```python
from build123d import *

# Parameters (mm, degrees)
F1_DEPTH = 1
F2_R     = 1.6
F3_DEPTH = 1.001
F4_R     = 0.5
F5_DEPTH = 1.001
F7_DEPTH = 1.001


with BuildPart() as f1:
    # F0 (on Front) → F1 (new body)
    with BuildSketch(Plane.XZ):
        Polygon((2, 30), (0, 30), (0, 0), (2, 0), (2, -1.3), (7, -1.3), (7, 0), (13, 0), (13, -1.3), (18, -1.3), (18, 0), (25, 0), (25, 30), (18, 30), (18, 31.3), (13, 31.3), (13, 30), (7, 30), (7, 31.3), (2, 31.3), align=None)
    extrude(amount=F1_DEPTH)

    # F2 (on face) → F3 (cut, through all)
    with BuildSketch(Plane.XZ.offset(1)):
        with Locations((10, 14)):
            Circle(F2_R)
        with BuildLine():
            ThreePointArc((13.328119, 21.137174), (17.755361, 15.367479), (15.568466, 8.431534))
            ThreePointArc((15.568466, 8.431534), (15.568466, 6.663767), (17.336233, 6.663767))
            ThreePointArc((17.336233, 6.663767), (20.21738, 15.8016), (14.384664, 23.402943))
            ThreePointArc((14.384664, 23.402943), (12.723507, 22.798331), (13.328119, 21.137174))
        make_face()
        with BuildLine():
            ThreePointArc((6.641243, 10.641243), (5.25, 14), (6.641243, 17.358757))
            ThreePointArc((6.641243, 17.358757), (6.641243, 19.126524), (4.873476, 19.126524))
            ThreePointArc((4.873476, 19.126524), (2.75, 14), (4.873476, 8.873476))
            ThreePointArc((4.873476, 8.873476), (6.641243, 8.873476), (6.641243, 10.641243))
        make_face()
    extrude(amount=-F3_DEPTH, mode=Mode.SUBTRACT)

    # F4 (on face) → F5 (cut, through all)
    with BuildSketch(Plane.XZ.offset(1)):
        with Locations((1.5, 30)):
            Circle(F4_R)
        with Locations((7.5, 30)):
            Circle(F4_R)
        with Locations((12.5, 30)):
            Circle(F4_R)
        with Locations((18.5, 30)):
            Circle(F4_R)
        with Locations((1.5, 0)):
            Circle(F4_R)
        with Locations((7.5, 0)):
            Circle(F4_R)
        with Locations((12.5, 0)):
            Circle(F4_R)
        with Locations((18.5, 0)):
            Circle(F4_R)
    extrude(amount=-F5_DEPTH, mode=Mode.SUBTRACT)

    # F6 (on face) → F7 (cut, through all)
    with BuildSketch(Plane.XZ.offset(1)):
        with BuildLine():
            Line((20, 0), (25, 0))
            Line((25, 0), (25, 30))
            Line((25, 30), (20, 30))
            Line((20, 30), (23.024917, 17.040091))
            ThreePointArc((23.024917, 17.040091), (23.372192, 13.725957), (22.88943, 10.428834))
            Line((22.88943, 10.428834), (20, 0))
        make_face()
    extrude(amount=-F7_DEPTH, mode=Mode.SUBTRACT)


solid = f1.part
```
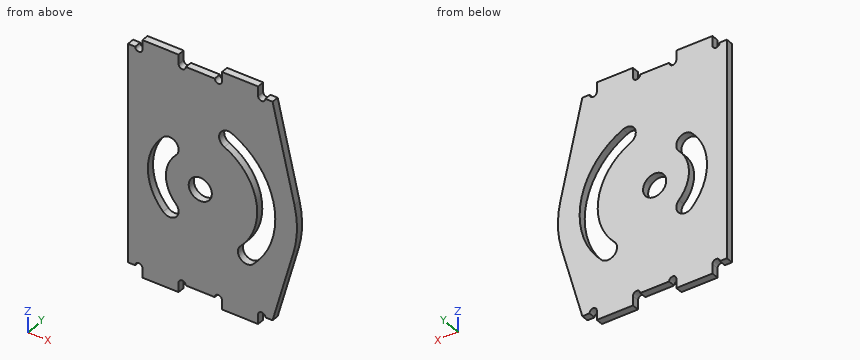
Check sheet for the modelled part. Datum: model origin and axes. Units: mm. Give positions to 0.01 mm unless a question says otherwise; leave off trailing zeros. Order: outer loops, then holes, each group sorted by start corner. A loop starts at its lowest first (then second) coordinate and runs counter-clockwise, first axis right, second up. Notation, with made-up numbers: M 83,40.25 L 116,40.25 A33 cw 116,79.25 Z; hole C 86.25,58 d3. An arc over 180 degrees is marked long. Answer in a Markdown table with one row per item.
1) Thickness scan on L1, parallel to Z at x = 10, y = -0.65; L2, parallel to X at y = -0.45, z = 9; L3, parallel to X at y = -0.25, z = 19. Record the ranges inside material, lowest first. Write a range as [from, to].
Filled sheet:
| item | result |
|---|---|
| L1 | z = [0, 12.4], [15.6, 30] |
| L2 | x = [0, 4.75], [6.75, 16.08], [19.09, 22.49] |
| L3 | x = [0, 4.75], [6.75, 16.08], [19.09, 22.57] |
2) Cross-section at C-C, the plane x = 18.5. Enter the section's corners in (y, z).
Filled sheet:
| item | result |
|---|---|
| outline | M -1,0.5 L 0,0.5 L 0,8.05 L -1,8.05 Z; M -1,19.95 L 0,19.95 L 0,29.5 L -1,29.5 Z |
3) Cross-section at D-D, the plane y = -0.5. Count the separate pieces of the cut face and the enclosed holes in it, plus the area to 3 significant figures.
Filled sheet:
| item | result |
|---|---|
| separate pieces | 1 |
| enclosed holes | 3 |
| area | 594 mm2 |
4) Gauge pin test, flat ends, axial feed: P1, Ø0.5, axis at x = 19.5, y = -0.5, coming from the +Z side; P2, Ø0.5, axis at y = -0.5, z = 31, coming from the +X side. Record the tip position at first contact, or that the pin passes through.
Filled sheet:
| item | result |
|---|---|
| P1 | stops at z = 30 |
| P2 | stops at x = 18 |
5) Cross-section at A-A, the plane x = 10. Enter the section's corners in (y, z).
Filled sheet:
| item | result |
|---|---|
| outline | M -1,0 L 0,0 L 0,12.4 L -1,12.4 Z; M -1,15.6 L 0,15.6 L 0,30 L -1,30 Z |
6) Cross-section at B-B, the plane z = 18. Enter the section's corners in (x, y), plus the area to 3 significant figures.
Filled sheet:
| item | result |
|---|---|
| outline | M 0,-1 L 3.95,-1 L 3.95,0 L 0,0 Z; M 6.98,-1 L 16.78,-1 L 16.78,0 L 6.98,0 Z; M 19.57,-1 L 22.8,-1 L 22.8,0 L 19.57,0 Z |
| area | 17.0 mm2 |
